```python
from build123d import *

# Parameters (mm, degrees)
SKETCH3_R          = 1.5
CUT_EXTRUDE1_DEPTH = 12.66190379
CIRPATTERN1_COUNT  = 2
CIRPATTERN1_ANGLE  = 135
CUT_EXTRUDE2_START = -0.5
SKETCH4_R          = 6
CUT_EXTRUDE2_DEPTH = 0.5


with BuildPart() as part:
    # Sketch2 → Revolve1 (revolve)
    with BuildSketch(Plane.XY, mode=Mode.PRIVATE) as revolve1_sk:
        with BuildLine():
            Line((6, 8), (4, 8))
            Line((4, 8), (4, -4))
            Line((4, -4), (6, -4))
            Line((6, -4), (6, -1.519868415))
            ThreePointArc((6, -1.519868415), (5.3, 0), (6, 1.519868415))
            Line((6, 1.519868415), (6, 4))
            Line((6, 4), (6, 8))
        make_face()
    revolve(revolve1_sk.sketch.rotate(Axis((0, 0, 0), (0, 1, 0)), 90), axis=Axis((0, 0, 0), (0, 1, 0)))

    # Sketch3 → Cut-Extrude1 (cut, through all)
    with BuildSketch(Plane.XY):
        with Locations(Location((0, 5.5, 0), (0, 0, 270.000000001))):
            Circle(SKETCH3_R)
    cut_extrude1 = extrude(amount=-CUT_EXTRUDE1_DEPTH, mode=Mode.SUBTRACT)

    # CirPattern1: Cut-Extrude1 ×2 about axis
    cirpattern1_axis = Axis((0, 8, 0), (0, -1, 0))
    for i in range(1, CIRPATTERN1_COUNT):
        add(cut_extrude1.rotate(cirpattern1_axis, i * CIRPATTERN1_ANGLE / (CIRPATTERN1_COUNT - 1)), mode=Mode.SUBTRACT)

    # Sketch4 → Cut-Extrude2 (cut)
    with BuildSketch(Plane.XZ.offset(4).offset(CUT_EXTRUDE2_START)):
        with Locations(Location((0, 0, 0), (0, 0, 270))):
            Circle(SKETCH4_R)
    extrude(amount=CUT_EXTRUDE2_DEPTH, mode=Mode.SUBTRACT)


solid = part.part
```
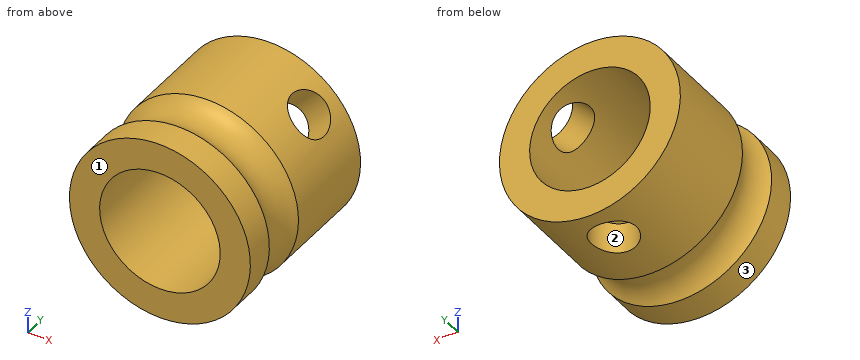
The model under review builds one solid part; all positions refer to its coordinate system, in mm. Face numbers are marked on the shaded views. Round coordinates to 2 decimals unless told otherwise and drop trailing zeros. Loops run counter-clockwise (first coordinate to the right, second up) from the corner with the lowest first, then second, coordinate; pieces in that order, holes last. Notation, with made-up numbers: (22, 81.5) - (32, 81.5) arc R23 ccw to (32, 92.5) - close; hole circle Ø11 at (59.5, 34). An arc over 180 degrees is marked (long way). Write each question's results on one line, items separated by ' | '. Start each with the question number.
Q1. Insertion check: P1, Ø3, axis at y = -1.5, z = -3.5, coming from the -X side; P2, Ø2, axis at y = 2, z = -3.5, coming from the -X side. Each pin has a flat end and moves straight along its axis. Give the tip position at first contact, or say it passes through.
Q2. Take a section at D-D on y = -1.75. Give the boundary of the cut face in (x, z), plus the area to 3 significant figures.
Q3. Wall thickness on line 1 along X through (y, z) = (2.25, 0); line 2 along Z through (x, y) = (0, 4.5); line 3 along Z through (x, y) = (-1, 2.5): over which ranges is each line inside the solid? List them lowest first. Write a range as [from, to].
Q4. Take a section at C-C on y = 4.75. Give the boundary of the cut face in (x, z), plus the area to 3 significant figures.
Q5. Take a section at B-B on z = 0. Give the boundary of the cut face in (x, y).
Q6. Draft analysis for pull direction Y (two halves, no side actions). For the marked faces 1, 2 and 3, state which applies: pulls with the +Y half, pulls with the -Y half, needs draft (parallel to the pull), parting line crosses it, or undercut.
Q7. Take a section at A-A on x = 0. Give the boundary of the cut face in (y, z).
Data:
1) P1: stops at x = -5.66 | P2: stops at x = -5.45
2) outline: circle Ø12 at (0, 0); hole circle Ø8 at (0, 0) | area: 62.8 mm²
3) line 1: x = [-6, -4], [4, 6] | line 2: z = [4, 6] | line 3: z = [-5.92, -3.87], [3.87, 5.92]
4) outline: (-1.3, -5.86) - (-1.3, -3.78) arc R4 cw (long way) to (1.76, 3.59) - (3.22, 5.06) arc R6 ccw (long way) to start; (1.3, -5.86) arc R6 ccw to (5.06, 3.22) - (3.59, 1.76) arc R4 cw to (1.3, -3.78) - close | area: 52.3 mm²
5) outline: (-6, -3.5) - (-4, -3.5) - (-4, 8) - (-6, 8) - (-6, 1.52) arc R2 cw to (-6, -1.52) - close; (4, -3.5) - (6, -3.5) - (6, -1.52) arc R2 cw to (6, 1.52) - (6, 8) - (4, 8) - close
6) face 1: pulls with the -Y half | face 2: undercut | face 3: needs draft
7) outline: (-3.5, -6) - (-1.52, -6) arc R2 cw to (1.52, -6) - (4, -6) - (4, -4) - (-3.5, -4) - close; (-3.5, 4) - (8, 4) - (8, 6) - (1.52, 6) arc R2 cw to (-1.52, 6) - (-3.5, 6) - close; (7, -6) - (8, -6) - (8, -4) - (7, -4) - close
